Can you work these out from the drawing? Everything is in mm from the part's minimum corner. Coordinates: 2 decimals unless noted, no trailing zeros. Write each loop counter-clockwise with the first axis right and the second up, starting at its lowest first coordinate (ties: lowest second). Pieces come first, ordered by that corner, then holes.
(1) Imagine slicing it at A-A, the plane z = 0.6. List the corners of the cut face in (x, y) for me (1 decimal).
(2) For pin 1 Ø0.8 at (y, z) = (49, 1) entering from -X, with a flat end and sliding along its axis, tell me the tip position at first contact or that it passes through.
(3) Please list where these lines run through material, in increasing order: probe 1 along Y at (x, z) = (27.5, 0.55) (1 decimal); probe 2 along X at (y, z) = (49, 0.15); probe 3 along Y at (x, z) = (3, 0.15).
(4) Imagine slicing it at B-B, the plane x = 3. List the corners of the cut face in (y, z) for me (1 decimal).
(5) Imagine slicing it at C-C, the plane x = 9.5. List the corners of the cut face in (y, z) for me (1 decimal).
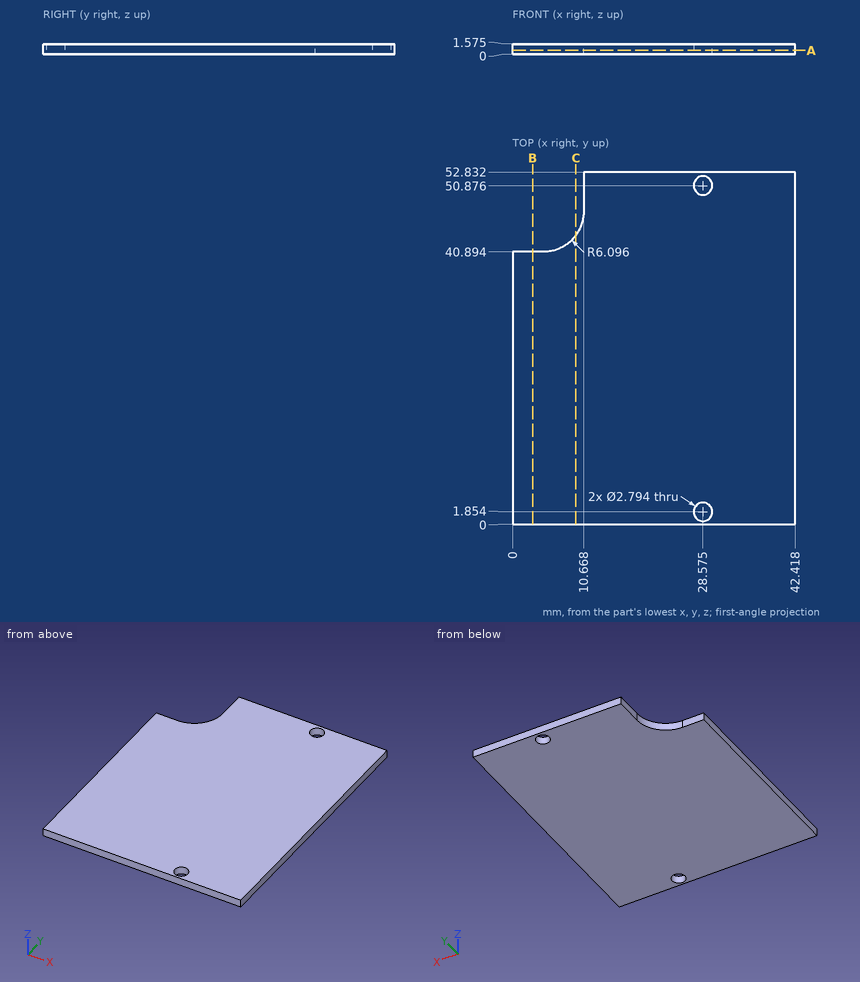
Recorded:
1. outline: (0, 0) - (42.4, 0) - (42.4, 52.8) - (10.7, 52.8) - (10.7, 47) arc R6.1 cw to (4.6, 40.9) - (0, 40.9) - close; hole circle Ø2.8 at (28.6, 1.9); hole circle Ø2.8 at (28.6, 50.9)
2. pin 1: stops at x = 10.67
3. probe 1: y = 0 to 1, 2.7 to 50, 51.8 to 52.8
3. probe 2: x = 10.67 to 42.42
3. probe 3: y = 0 to 40.89
4. outline: (0, 0) - (40.9, 0) - (40.9, 1.6) - (0, 1.6) - close
5. outline: (0, 0) - (43.4, 0) - (43.4, 1.6) - (0, 1.6) - close
